Build history of the part. All positions in model axes, mm. Face numbers are marked on the shaded views. A direction names the side the tool comes from. Coordinates: 2 decimals unless noted, no trailing zeros. Order: outer loops, then holes, each group sorted by start corner. A loop starts at its lowest first (then second) coordinate and runs counter-clockwise, first axis right, second up. Notation, with made-up numbers: (38, 52.25) - (45, 52.25) arc R9 cw to (45, 64.25) - close; hole circle Ø11 at (78, 26.5). An arc over 180 degrees is marked (long way). Return JSON: item names as keys, results as strings.
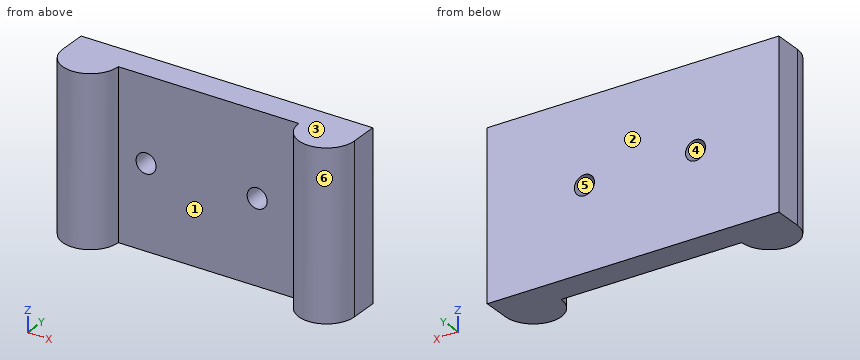
Autodesk Inventor part; units mm, degrees
ref_plane "YZ Plane" through (0, 0, 0) normal (1, 0, 0) x (0, 1, 0)
ref_plane "XZ Plane" through (0, 0, 0) normal (0, 1, 0) x (-1, 0, 0)
ref_plane "XY Plane" through (0, 0, 0) normal (0, 0, 1) x (1, 0, 0)
sketch "Sketch1" plane through (0, 0, 0) normal (0, 0, 1) x (1, 0, 0)
  line L0 (-48.1538, -4.158) -> (-48.1538, 2.192)
  line L1 (-48.1538, 2.192) -> (18.5212, 2.192)
  line L2 (18.5212, 2.192) -> (18.5212, -4.158)
  arc A0 (5.8212, -4.158) -> (18.5212, -4.158) centre (12.1712, -4.158) ccw
  line L3 (5.8212, -4.158) -> (-35.4538, -4.158)
  arc A1 (-48.1538, -4.158) -> (-35.4538, -4.158) centre (-41.8038, -4.158) ccw
  dimension "d0" = 6.35
  dimension "d1" = 6.35
  dimension "d2" = 66.675
extrude "Extrusion1" add sketch "Sketch1" along normal blind 38.1
sketch "Sketch2" plane through (-48.1538, 2.192, 0) normal (0, 1, 0) x (1, 0, 0)
  line L0 (0, 0) -> (0, -38.1)
  line L1 (19.05, -19.05) -> (44.45, -19.05)
  point P0 (66.675, 0)
  dimension "d5" = 22.225
  dimension "d6" = 25.4
  dimension "d7" = 19.05
hole "Hole1" at (-3.7038, 2.192, 19.05) at (-29.1038, 2.192, 19.05) direction (0, -1, 0) diameter 4.572 end through all
properties part number "locator"
1. Tool access for the marked faces 1 and 2: list every direction of +Z, -Z, +X, -X, +Y, -Y with a clear straight run to the whole face (end or side of a thin tool).
Check values:
{"face 1": "+Z, -Z, -Y", "face 2": "+Z, -Z, +X, -X, +Y"}
2. Cut at D-D on x = -26. Give the cut face in (y, z).
Check values:
{"outline": "(-4.16, 0) - (2.19, 0) - (2.19, 38.1) - (-4.16, 38.1) - close"}
3. Cut at B-B on x = -2.5. Give the cut face in (y, z), plus the area to 3 significant figures.
Check values:
{"outline": "(-4.16, 0) - (2.19, 0) - (2.19, 17.11) - (-4.16, 17.11) - close; (-4.16, 20.99) - (2.19, 20.99) - (2.19, 38.1) - (-4.16, 38.1) - close", "area": "217 mm²"}
4. Probe L1, parallel to X at y = -0.5, z = 19.05; L2, parallel to Y at x = 1, z = 10.5; L3, parallel to Z at x = -30, y = -4. List the from-to ranges inside material, lowest first.
Check values:
{"L1": "-48.15 to -31.39, -26.82 to -5.99, -1.42 to 18.52", "L2": "-4.16 to 2.19", "L3": "0 to 16.95, 21.15 to 38.1"}
5. Cut at A-A on z = 19.05. Give the cut face in (x, y).
Check values:
{"outline": "(-48.15, -4.16) arc R6.35 ccw to (-35.45, -4.16) - (-31.39, -4.16) - (-31.39, 2.19) - (-48.15, 2.19) - close; (-26.82, -4.16) - (-5.99, -4.16) - (-5.99, 2.19) - (-26.82, 2.19) - close; (-1.42, -4.16) - (5.82, -4.16) arc R6.35 ccw to (18.52, -4.16) - (18.52, 2.19) - (-1.42, 2.19) - close"}
6. Drop flat-ended pins along their axis: pin 1 (6 mm diameter, centred on x = -29.1, z = 19.05, fed in from -Y); pin 2 (1 mm diameter, centred on y = -7.5, z = 11, fed in from -X); pin 3 (2 mm diameter, centred on y = -6.5, z = 17, fed in from +X). Give the stop position or say it passes through.
Check values:
{"pin 1": "y = -4.16", "pin 2": "x = -47.48", "pin 3": "x = 18.38"}
7. Cut at C-C on z = 7. Give the cut face in (x, y), plus the area to 3 significant figures.
Check values:
{"outline": "(-48.15, -4.16) arc R6.35 ccw to (-35.45, -4.16) - (5.82, -4.16) arc R6.35 ccw to (18.52, -4.16) - (18.52, 2.19) - (-48.15, 2.19) - close", "area": "550 mm²"}
8. Mould opens along Z. For the marked faces 3, 4, 5 and 6 say: pulls with the +Z half, pulls with the -Z half, needs draft (parallel to the pull), parting line crosses it, or undercut.
Check values:
{"face 3": "pulls with the +Z half", "face 4": "undercut", "face 5": "undercut", "face 6": "needs draft"}
